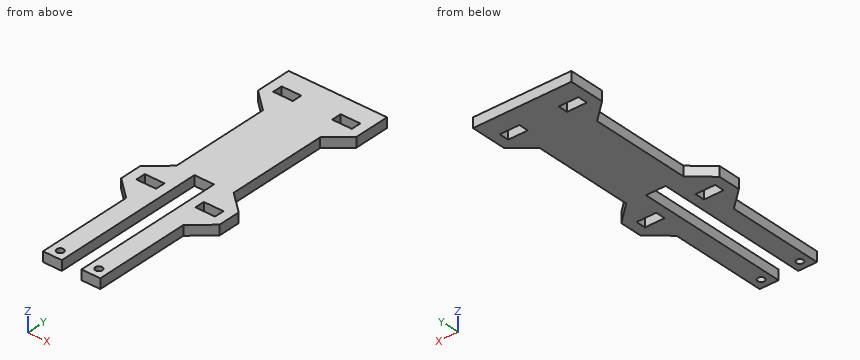
from build123d import *

# Parameters (mm, degrees)
SKETCH1_R           = 2.1
SKETCH1_W           = 12
SKETCH1_H           = 6
BOSS_EXTRUDE1_DEPTH = 6


with BuildPart() as part:
    # Sketch1 → Boss-Extrude1 (new body)
    with BuildSketch(Plane.XY):
        Polygon((24.958587154, 66.332129581), (-35.041412846, 66.332129581), (-35.041412846, 44.514954247), (-22.5134665, 33.454149031), (-22.5134665, -28.072174919), (-35.041412846, -39.132980135), (-35.041412846, -52.767330805), (-22.5134665, -63.828136021), (-22.5134665, -122.961056524), (-11.041412846, -122.961056524), (-11.041412846, -73.667870419), (-11.041412846, -28.667870419), (0.958587154, -28.667870419), (0.958587154, -73.667870419), (0.958587154, -122.961056524), (12.430640807, -122.961056524), (12.430640807, -63.828136021), (24.958587154, -52.767330805), (24.958587154, -39.132980135), (12.430640807, -28.072174919), (12.430640807, 33.454149031), (24.958587154, 44.514954247), align=None)
        with Locations((-16.777439673, -117.386123735)):
            Circle(SKETCH1_R, mode=Mode.SUBTRACT)
        with Locations((-23.041412846, -45.95015547)):
            Rectangle(SKETCH1_W, SKETCH1_H, mode=Mode.SUBTRACT)
        with Locations((6.69461398, -117.276997452)):
            Circle(SKETCH1_R, mode=Mode.SUBTRACT)
        with Locations((12.958587154, -45.95015547)):
            Rectangle(SKETCH1_W, SKETCH1_H, mode=Mode.SUBTRACT)
        with Locations((-23.041412846, 51.332129581)):
            Rectangle(SKETCH1_W, SKETCH1_H, mode=Mode.SUBTRACT)
        with Locations((12.958587154, 51.332129581)):
            Rectangle(SKETCH1_W, SKETCH1_H, mode=Mode.SUBTRACT)
    extrude(amount=BOSS_EXTRUDE1_DEPTH)


solid = part.part
Can you work these out from the model? Positions are in its coordinate system, mm. Coordinates: 2 decimals unless noted, no trailing zeros. Loops run counter-clockwise (first coordinate to the right, second up) from the corner with the lowest first, then second, coordinate; pieces in that order, holes last. Notation, with made-up numbers: (14.25, 60) - (71.25, 60) arc R16 ccw to (71.25, 89) - close; hole circle Ø7 at (38, -29.5). An arc over 180 degrees is marked (long way). Answer as a JSON object with one key per item and string values. Group by question number.
Item 1: If we section it at D-D (z = 1.9): State how many separate pieces and enclosed holes the cut face has, plus the area to 3 significant figures.
Item 2: If we section it at C-C (y = 13): List the corners of the cut face in (x, z) for me, plus the area to 3 significant figures.
Item 3: If I drill on L1, parallel to Y at x = 11, z = 1.9; L2, parallel to X at y = -78.5, z = 1.7; L3, parallel to Y at x = -24.5, z = 1.15, over which ranges is the centre line in solid material (lowest first)? Write a range as from..to.
Item 4: If we section it at A-A (y = -84.5): List the corners of the cut face in (x, z) for me.
Item 5: If we section it at B-B (x = 21.5): List the corners of the cut face in (y, z) for me.
Item 6: For pin 1 (2 mm diameter, centred on y = -79, z = 1, fed in from -X); pin 2 (1.8 mm diameter, centred on x = -24.5, z = 1.5, fed in from -Y), each with a flat end and sliding along its axis, tell me the tip position at first contact or that it passes through.
Returned:
{
 "1": {"separate pieces": "1", "enclosed holes": "6", "area": "6,470 mm²"},
 "2": {"outline": "(-22.51, 0) - (12.43, 0) - (12.43, 6) - (-22.51, 6) - close", "area": "210 mm²"},
 "3": {"L1": "y = -122.96..-48.95, -42.95..48.33, 54.33..66.33", "L2": "x = -22.51..-11.04, 0.96..12.43", "L3": "y = -62.07..-48.95, -42.95..-29.83, 35.21..48.33, 54.33..66.33"},
 "4": {"outline": "(-22.51, 0) - (-11.04, 0) - (-11.04, 6) - (-22.51, 6) - close; (0.96, 0) - (12.43, 0) - (12.43, 6) - (0.96, 6) - close"},
 "5": {"outline": "(-55.82, 0) - (-36.08, 0) - (-36.08, 6) - (-55.82, 6) - close; (41.46, 0) - (66.33, 0) - (66.33, 6) - (41.46, 6) - close"},
 "6": {"pin 1": "stops at x = -22.51", "pin 2": "stops at y = -62.87"}
}
